from build123d import *

# Parameters (mm, degrees)
SKETCH1_R           = 2
BOSS_EXTRUDE1_DEPTH = 2.54
SKETCH2_W           = 8.89
SKETCH2_H           = 3.81
BOSS_EXTRUDE2_DEPTH = 7.62


with BuildPart() as part:
    # Sketch1 → Boss-Extrude1 (new body)
    # profile 1 of 2: a face of its own
    with BuildSketch(Plane.XY):
        with BuildLine():
            ThreePointArc((42.939465347, 5.941095032), (41.487522441, 5.056745133), (40.918582885, 3.454708702))
            Line((40.918582885, 3.454708702), (40.918582885, 3.15450519))
            Line((40.918582885, 3.15450519), (40.918582885, -15.00649481))
            Line((40.918582885, -15.00649481), (40.918582885, -19.15304481))
            ThreePointArc((40.918582885, -19.15304481), (40.174634109, -20.949096034), (38.378582885, -21.69304481))
            Line((38.378582885, -21.69304481), (-2.034570627, -21.69304481))
            ThreePointArc((-2.034570627, -21.69304481), (-3.636607058, -22.261984366), (-4.520956957, -23.713927272))
            ThreePointArc((-4.520956957, -23.713927272), (-12.957358938, -26.229486634), (-10.441799577, -17.793084652))
            ThreePointArc((-10.441799577, -17.793084652), (-8.989856671, -16.908734753), (-8.420917115, -15.306698322))
            Line((-8.420917115, -15.306698322), (-8.420917115, -14.63819481))
            Line((-8.420917115, -14.63819481), (-8.420917115, 2.78620519))
            Line((-8.420917115, 2.78620519), (-8.420917115, 7.30105519))
            ThreePointArc((-8.420917115, 7.30105519), (-7.676968339, 9.097106414), (-5.880917115, 9.84105519))
            Line((-5.880917115, 9.84105519), (34.532236397, 9.84105519))
            ThreePointArc((34.532236397, 9.84105519), (36.134272828, 10.409994746), (37.018622727, 11.861937652))
            ThreePointArc((37.018622727, 11.861937652), (45.455024709, 14.377497013), (42.939465347, 5.941095032))
        make_face()
        with Locations((-9.419138026, -22.691265722)):
            Circle(SKETCH1_R, mode=Mode.SUBTRACT)
        with Locations((41.916803797, 10.839276102)):
            Circle(SKETCH1_R, mode=Mode.SUBTRACT)
        with BuildLine():
            ThreePointArc((38.378582885, 6.03105519), (38.006608497, 6.929080802), (37.108582885, 7.30105519))
            Line((37.108582885, 7.30105519), (-4.610917115, 7.30105519))
            ThreePointArc((-4.610917115, 7.30105519), (-5.508942727, 6.929080802), (-5.880917115, 6.03105519))
            Line((-5.880917115, 6.03105519), (-5.880917115, 2.78620519))
            Line((-5.880917115, 2.78620519), (-5.880917115, -14.63819481))
            Line((-5.880917115, -14.63819481), (-5.880917115, -17.88304481))
            ThreePointArc((-5.880917115, -17.88304481), (-5.508942727, -18.781070422), (-4.610917115, -19.15304481))
            Line((-4.610917115, -19.15304481), (37.108582885, -19.15304481))
            ThreePointArc((37.108582885, -19.15304481), (38.006608497, -18.781070422), (38.378582885, -17.88304481))
            Line((38.378582885, -17.88304481), (38.378582885, -15.00649481))
            Line((38.378582885, -15.00649481), (38.378582885, 3.15450519))
            Line((38.378582885, 3.15450519), (38.378582885, 6.03105519))
        make_face(mode=Mode.SUBTRACT)
    # profile 2 of 2: a face of its own
    with BuildSketch(Plane.XY):
        with BuildLine():
            Line((38.378582885, 6.03105519), (38.378582885, 3.15450519))
            Line((38.378582885, 3.15450519), (38.378582885, -15.00649481))
            Line((38.378582885, -15.00649481), (38.378582885, -17.88304481))
            ThreePointArc((38.378582885, -17.88304481), (38.006608497, -18.781070422), (37.108582885, -19.15304481))
            Line((37.108582885, -19.15304481), (-4.610917115, -19.15304481))
            ThreePointArc((-4.610917115, -19.15304481), (-5.508942727, -18.781070422), (-5.880917115, -17.88304481))
            Line((-5.880917115, -17.88304481), (-5.880917115, -14.63819481))
            Line((-5.880917115, -14.63819481), (-5.880917115, 2.78620519))
            Line((-5.880917115, 2.78620519), (-5.880917115, 6.03105519))
            ThreePointArc((-5.880917115, 6.03105519), (-5.508942727, 6.929080802), (-4.610917115, 7.30105519))
            Line((-4.610917115, 7.30105519), (37.108582885, 7.30105519))
            ThreePointArc((37.108582885, 7.30105519), (38.006608497, 6.929080802), (38.378582885, 6.03105519))
        make_face()
    extrude(amount=BOSS_EXTRUDE1_DEPTH)

    # Sketch2 → Boss-Extrude2 (add)
    with BuildSketch(Plane.XY.offset(2.54)):
        with BuildLine():
            Line((31.613029704, -21.69304481), (31.613029704, -25.50304481))
            add(Edge.make_bspline(
                [(31.613029704, -25.50304481), (32.285115867, -25.50304481), (32.316518426, -22.279360341), (33.645471093, -21.69304481)],
                knots=[0, 0, 0, 0, 1, 1, 1, 1], degree=3))
            Line((33.645471093, -21.69304481), (31.613029704, -21.69304481))
        make_face()
        with BuildLine():
            add(Edge.make_bspline(
                [(22.723029704, -25.50304481), (22.050943542, -25.50304481), (22.019540983, -22.279360341), (20.690588316, -21.69304481)],
                knots=[0, 0, 0, 0, 1, 1, 1, 1], degree=3))
            Line((22.723029704, -25.50304481), (22.723029704, -21.69304481))
            Line((22.723029704, -21.69304481), (20.690588316, -21.69304481))
        make_face()
        with Locations((27.168029704, -23.59804481)):
            Rectangle(SKETCH2_W, SKETCH2_H)
        with BuildLine():
            Line((20.690588316, 9.84105519), (22.723029704, 9.84105519))
            Line((22.723029704, 9.84105519), (22.723029704, 13.65105519))
            add(Edge.make_bspline(
                [(22.723029704, 13.65105519), (22.050943542, 13.65105519), (22.019540983, 10.427370721), (20.690588316, 9.84105519)],
                knots=[0, 0, 0, 0, 1, 1, 1, 1], degree=3))
        make_face()
        with Locations((27.168029704, 11.74605519)):
            Rectangle(SKETCH2_W, SKETCH2_H)
        with BuildLine():
            Line((31.613029704, 13.65105519), (31.613029704, 9.84105519))
            Line((31.613029704, 9.84105519), (33.645471093, 9.84105519))
            add(Edge.make_bspline(
                [(31.613029704, 13.65105519), (32.285115867, 13.65105519), (32.316518426, 10.427370721), (33.645471093, 9.84105519)],
                knots=[0, 0, 0, 0, 1, 1, 1, 1], degree=3))
        make_face()
    extrude(amount=-BOSS_EXTRUDE2_DEPTH)


solid = part.part
For this review, take the finished solid that the model builds, in its own axes (mm). A direction names the side the tool comes from. Round coordinates to 2 decimals unless told otherwise and drop trailing zeros. Order: outer loops, then holes, each group sorted by start corner. A loop starts at its lowest first (then second) coordinate and runs counter-clockwise, first axis right, second up. Notation, with made-up numbers: M 5.5,-22.5 L 50.5,-22.5 A26 ccw 50.5,4.5 Z; hole C 67.5,9 d1. An arc over 180 degrees is marked long. Use a Markdown table: item, result. Add a question column.
Item 1: Add section C-C, the plane y = -17. Give the boundary of the cut face in (x, z).
Item 2: Tool access review of faces 5 (the flat face through (36, -21.693, 1)), 6 (the cylindrical face through (-3.62, -22.25, 1.25)), 7 (the cylindrical face through (36.115, 10.395, 1.252)), 8 (the flat face through (7, 9.841, 1)), 9 (the flat face through (16, -6, 2.54)): name each direction out of +Z, -Z, +X, -X, +Y, -Y from which nothing blocks a thin tool from reaching the whole face with its end or side.
Item 3: Add section A-A, the plane z = 0.75. State how many separate pieces and enclosed holes the cut face has, then the cut area to 3 significant figures.
Item 4: To check wall thickness, follow line 1 along Y through (x, z) = (28.5, -1.75); line 2 along X through (y, z) = (-6, 0.5); line 3 along Y through (x, z) = (34.5, 2). State the ranges of each line that lie inside material, in increasing order.
Item 5: Mouldability with a two-part tool opening along Y and no side actions: class faces 1 (the flat face through (27, 13.651, -1)), 2 (the flat face through (27, 9.841, -3)), 3 (the cylindrical face through (39.92, 10.93, 1.25)), 4 (the flat face through (27, -25.503, -1)) as released by +Y, released by -Y, zero draft, split by the parting line, or undercut.
Item 6: Insertion check: pin 1 (2 mm diameter, centred on x = 7.5, z = 1.5, fed in from -Y); pin 2 (2 mm diameter, centred on x = 31, y = -17.5, fed in from -Z); pin 3 (3 mm diameter, centred on x = 6, z = 0.5, fed in from +Y). Each pin has a flat end and moves straight along its axis. Give the tip position at first contact, or say it passes through.
Item 7: Add section B-B, the plane x = 17. Give the boundary of the cut face in (y, z), then the cut area to 3 significant figures.
Geometry results:
| question | item | result |
|---|---|---|
| 1 | outline | M -9.07,0 L 40.92,0 L 40.92,2.54 L -9.07,2.54 Z |
| 2 | face 5 | +Z, -Z, +X, -Y |
| 2 | face 6 | +Z, -Z, -Y |
| 2 | face 7 | +Z, -Z, +Y |
| 2 | face 8 | +Z, -Z, -X, +Y |
| 2 | face 9 | +Z, +X, -X, +Y, -Y |
| 3 | separate pieces | 1 |
| 3 | enclosed holes | 2 |
| 3 | area | 1,750 mm² |
| 4 | line 1 | y = -25.5 to -21.69, 9.84 to 13.65 |
| 4 | line 2 | x = -8.42 to 40.92 |
| 4 | line 3 | y = -21.69 to 9.84 |
| 5 | face 1 | released by +Y |
| 5 | face 2 | undercut |
| 5 | face 3 | undercut |
| 5 | face 4 | released by -Y |
| 6 | pin 1 | stops at y = -21.69 |
| 6 | pin 2 | stops at z = 0 |
| 6 | pin 3 | stops at y = 9.84 |
| 7 | outline | M -21.69,0 L 9.84,0 L 9.84,2.54 L -21.69,2.54 Z |
| 7 | area | 80.1 mm² |
